from build123d import *

# Parameters (mm, degrees)
SKETCH_1_R      = 5
EXTRUDE_3_DEPTH = 0.1


with BuildPart() as part:
    # 草图1 → 凸台-拉伸3 (new body)
    with BuildSketch(Plane.XY):
        Circle(SKETCH_1_R)
        Polygon((-0.167777112, -1.005793851), (1.720384349, -1.005793851), (1.788940866, -1.005793851), (2.645033635, -3.640576475), (0, -1.718847051), (-2.645033635, -3.640576475), (-1.788940866, -1.005793851), (-1.196984608, -1.005793851), (-1.064898778, -1.005793851), (-1.045698937, -0.805793851), (-0.898132968, -0.805793851), (-0.880039365, -0.617317259), (-0.305168214, -0.766751199), (-0.308916278, -0.805793851), (-0.167777112, -0.805793851), align=None, mode=Mode.SUBTRACT)
        with BuildLine():
            Line((-1.991956336, 0.60790071), (-1.899072205, 0.644948492))
            add(Edge.make_bspline(
                [(-1.899072205, 0.644948492), (-1.780698643, 0.348168911), (-1.304567249, -0.127672291), (-0.336736042, -0.504525958), (0.252920379, -0.581061249), (0.729572204, -0.501330005), (1.026706033, -0.397504088), (1.163445675, -0.341657163)],
                knots=[0, 0, 0, 0, 0.25, 0.5, 0.75, 0.875, 1, 1, 1, 1], degree=3))
            Line((1.163445675, -0.341657163), (1.201255585, -0.434233676))
            Line((1.201255585, -0.434233676), (1.239065495, -0.526810188))
            add(Edge.make_bspline(
                [(-2.084840467, 0.570852927), (-1.951454553, 0.236435213), (-1.399816024, -0.313391075), (-0.398090532, -0.695067628), (0.253747942, -0.784974301), (0.784004358, -0.694588239), (1.094323827, -0.585925285), (1.239065495, -0.526810188)],
                knots=[0, 0, 0, 0, 0.25, 0.5, 0.75, 0.875, 1, 1, 1, 1], degree=3))
            Line((-2.084840467, 0.570852927), (-1.991956336, 0.60790071))
        make_face(mode=Mode.SUBTRACT)
        Polygon((-4.279754323, 1.390576475), (-2.15, 1.390576475), (-2.15, -0.066596805), (-2.15, -0.156780615), align=None, mode=Mode.SUBTRACT)
        with BuildLine():
            add(Edge.make_bspline(
                [(-1.549830374, 0.538301968), (-1.367834784, 0.350062034), (-0.953039741, 0.039850566), (-0.14913383, -0.273116302), (0.644284758, -0.303181598), (1.121216686, -0.059789278), (1.302628316, 0.116501809)],
                knots=[0, 0, 0, 0, 0.25, 0.5, 0.75, 1, 1, 1, 1], degree=3))
            Line((1.302628316, 0.116501809), (1.372319625, 0.044786249))
            Line((1.372319625, 0.044786249), (1.442010933, -0.026929311))
            add(Edge.make_bspline(
                [(-1.693616475, 0.399285576), (-1.497925898, 0.196880775), (-1.049647981, -0.137319606), (-0.197096293, -0.473093583), (0.540683467, -0.49628987), (1.08406545, -0.311067402), (1.334925603, -0.130992039), (1.442010933, -0.026929311)],
                knots=[0, 0, 0, 0, 0.25, 0.5, 0.75, 0.875, 1, 1, 1, 1], degree=3))
            Line((-1.693616475, 0.399285576), (-1.621723425, 0.468793772))
            Line((-1.621723425, 0.468793772), (-1.549830374, 0.538301968))
        make_face(mode=Mode.SUBTRACT)
        with BuildLine():
            ThreePointArc((-0.840281876, 0.990576475), (-0.862451255, 1.000387117), (-0.870098497, 1.023392545))
            Line((-0.870098497, 1.023392545), (-0.856649718, 1.163485148))
            ThreePointArc((-0.856649718, 1.163485148), (-0.846976154, 1.182792155), (-0.826833098, 1.190576475))
            Line((-0.826833098, 1.190576475), (0.640511551, 1.190576475))
            ThreePointArc((0.640511551, 1.190576475), (0.787174219, 1.126554641), (0.839940758, 0.975477093))
            Line((0.839940758, 0.975477093), (0.812895447, 0.618268761))
            ThreePointArc((0.812895447, 0.618268761), (0.803392481, 0.598564726), (0.783027236, 0.590576475))
            Line((0.783027236, 0.590576475), (0.642533668, 0.590576475))
            ThreePointArc((0.642533668, 0.590576475), (0.620568222, 0.600164928), (0.612665457, 0.622791584))
            Line((0.612665457, 0.622791584), (0.617880458, 0.691670133))
            Line((0.617880458, 0.691670133), (0.624225734, 0.775477093))
            ThreePointArc((0.624225734, 0.775477093), (0.571459194, 0.926554641), (0.424796526, 0.990576475))
            Line((0.424796526, 0.990576475), (0.185889669, 0.990576475))
            Line((0.185889669, 0.990576475), (-0.136466154, 0.990576475))
            Line((-0.136466154, 0.990576475), (-0.174865836, 0.590576475))
            ThreePointArc((-0.174865836, 0.590576475), (-0.186605785, 0.569554584), (-0.210026076, 0.563965642))
            Line((-0.210026076, 0.563965642), (-0.730009604, 0.658240899))
            ThreePointArc((-0.730009604, 0.658240899), (-0.748550248, 0.669637431), (-0.754482606, 0.690576475))
            Line((-0.754482606, 0.690576475), (-0.725682844, 0.990576475))
            Line((-0.725682844, 0.990576475), (-0.840281876, 0.990576475))
        make_face(mode=Mode.SUBTRACT)
        Polygon((-1.010312947, 1.390576475), (0, 4.5), (1.010312947, 1.390576475), align=None, mode=Mode.SUBTRACT)
        with BuildLine():
            Line((-1.233981014, 0.474718903), (-1.175156308, 0.55558703))
            add(Edge.make_bspline(
                [(-1.175156308, 0.55558703), (-0.993921308, 0.423753933), (-0.60253903, 0.216218799), (0.110209984, 0.046440521), (0.771586805, 0.108296918), (1.136324529, 0.363638938), (1.265061247, 0.529994773)],
                knots=[0, 0, 0, 0, 0.25, 0.5, 0.75, 1, 1, 1, 1], degree=3))
            Line((1.265061247, 0.529994773), (1.344146249, 0.468793772))
            Line((1.344146249, 0.468793772), (1.423231251, 0.407592771))
            add(Edge.make_bspline(
                [(-1.29280572, 0.393850776), (-1.097129026, 0.251512571), (-0.673598325, 0.026850492), (0.090771832, -0.155398634), (0.834150505, -0.091874662), (1.271541178, 0.21157621), (1.423231251, 0.407592771)],
                knots=[0, 0, 0, 0, 0.25, 0.5, 0.75, 1, 1, 1, 1], degree=3))
            Line((-1.29280572, 0.393850776), (-1.233981014, 0.474718903))
        make_face(mode=Mode.SUBTRACT)
        with BuildLine():
            add(Edge.make_bspline(
                [(-0.824987307, 0.653212382), (-0.652216888, 0.565882813), (-0.294799178, 0.437574506), (0.340946716, 0.364657013), (0.791001776, 0.488979802), (1.051442622, 0.706562479), (1.151632496, 0.882886074), (1.184898576, 0.972197324)],
                knots=[0, 0, 0, 0, 0.25, 0.5, 0.75, 0.875, 1, 1, 1, 1], degree=3))
            Line((1.184898576, 0.972197324), (1.2786091, 0.937292631))
            Line((1.2786091, 0.937292631), (1.372319625, 0.902387938))
            add(Edge.make_bspline(
                [(-0.915209687, 0.474718903), (-0.728178948, 0.380181227), (-0.341272237, 0.241351144), (0.346598042, 0.160979838), (0.87745692, 0.299632533), (1.209299978, 0.577219377), (1.331357393, 0.792414409), (1.372319625, 0.902387938)],
                knots=[0, 0, 0, 0, 0.25, 0.5, 0.75, 0.875, 1, 1, 1, 1], degree=3))
            Line((-0.915209687, 0.474718903), (-0.870098497, 0.563965642))
            Line((-0.870098497, 0.563965642), (-0.824987307, 0.653212382))
        make_face(mode=Mode.SUBTRACT)
        Polygon((4.279754323, 1.390576475), (2, -0.265761995), (2, -0.022653284), (2, 1.390576475), align=None, mode=Mode.SUBTRACT)
    extrude(amount=EXTRUDE_3_DEPTH)


solid = part.part
Design review of the part built by this model. Coordinates are the model's own, in mm. Coordinates: 2 decimals unless noted, no trailing zeros. Loops run counter-clockwise (first coordinate to the right, second up) from the corner with the lowest first, then second, coordinate; pieces in that order, holes last.
Item 1: Clearance check with a flat-ended pin moving along its axis: pin 1 (4 mm diameter, centred on x = -0.5, y = -1, fed in from +Z). State where the tip first meets the part, or that it passes through.
Completed:
pin 1: stops at z = 0.1
Item 2: Add section D-D (x = 3.25). Write out the cut boundary in (y, z).
Completed:
outline: (-3.8, 0) - (0.64, 0) - (0.64, 0.1) - (-3.8, 0.1) - close; (1.39, 0) - (3.8, 0) - (3.8, 0.1) - (1.39, 0.1) - close
Item 3: Add section B-B (y = -1.5). Write out the cut boundary in (x, z).
Completed:
outline: (-4.77, 0) - (-1.95, 0) - (-1.95, 0.1) - (-4.77, 0.1) - close; (1.95, 0) - (4.77, 0) - (4.77, 0.1) - (1.95, 0.1) - close
Item 4: Add section C-C (y = -3.5). Write out the cut boundary in (x, z), and give its area (3 significant figures).
Completed:
outline: (-3.57, 0) - (-2.6, 0) - (-2.6, 0.1) - (-3.57, 0.1) - close; (-2.45, 0) - (2.45, 0) - (2.45, 0.1) - (-2.45, 0.1) - close; (2.6, 0) - (3.57, 0) - (3.57, 0.1) - (2.6, 0.1) - close
area: 0.685 mm2
Item 5: Add section A-A (x = -2.5). Write out the cut boundary in (y, z), and give its area (3 significant figures).
Completed:
outline: (-4.33, 0) - (-3.54, 0) - (-3.54, 0.1) - (-4.33, 0.1) - close; (-3.19, 0) - (0.1, 0) - (0.1, 0.1) - (-3.19, 0.1) - close; (1.39, 0) - (4.33, 0) - (4.33, 0.1) - (1.39, 0.1) - close
area: 0.703 mm2
Item 6: Wall thickness on L1, parallel to X at y = -1.25, z = 0.05; L2, parallel to X at y = 2.75, z = 0.05: over which ranges is each line inside the solid? List them lowest first.
Completed:
L1: x = -4.84 to -1.87, 1.87 to 4.84
L2: x = -4.18 to -0.57, 0.57 to 4.18
